from build123d import *

# Parameters (mm, degrees)
F0_R     = 21.2725
F1_DEPTH = 3.175
F2_R     = 21.2725
F3_DEPTH = 3.175
F4_R     = 11.43
F5_DEPTH = 0.889
F6_R     = 0.635


with BuildPart() as f1:
    # F0 (on Top) → F1 (new body)
    with BuildSketch(Plane.XY):
        Circle(F0_R)
    extrude(amount=-F1_DEPTH)

    # F2 (on face) → F3 (join)
    with BuildSketch(Plane(origin=(0, 0, -3.175), x_dir=(1, 0, 0), z_dir=(0, 0, -1))):
        Circle(F2_R)
    extrude(amount=F3_DEPTH)

    # F4 (on face) → F5 (join)
    with BuildSketch(Plane(origin=(0, 0, -6.35), x_dir=(1, 0, 0), z_dir=(0, 0, -1))):
        Circle(F4_R)
    extrude(amount=F5_DEPTH)

    # F6
    f6_edges = [f1.edges().sort_by_distance(p)[0] for p in [
        (-11.43, 0, -7.239),
    ]]
    fillet(f6_edges, radius=F6_R)


solid = f1.part
Geometry check sheet. Reference: the model listing, model coordinates, mm. A direction names the side the tool comes from. Coordinates: 2 decimals unless noted, no trailing zeros. Order: outer loops, then holes, each group sorted by start corner. A loop starts at its lowest first (then second) coordinate and runs counter-clockwise, first axis right, second up. Notation, with made-up numbers: (28, 30.25) -> (62, 30.25) arc R23 cw to (62, 47.25) -> close; hole circle Ø1 at (2, 25). An arc over 180 degrees is marked (long way). Use a Markdown table: item, result. Add a question column.
1. Cross-section at C-C (z = -3.5). Enter the section's corners in (x, y) (1 decimal).
2. Cross-section at D-D (x = -16.5). Enter the section's corners in (y, z).
3. Go/stop test with flat-tipped pins: pin 1 Ø1.5 at (x, z) = (8.5, -2.5) entering from -Y; pin 2 Ø2 at (y, z) = (5.5, -1.5) entering from -X; pin 3 Ø3 at (x, z) = (0.5, -1) entering from +Y. Record where each tip stops, or that it passes through.
4. Set-up check for faces 1 (the face through (9, 9, -6.35)), 2 (the face through (0, 0, 0)): record each of +Z, -Z, +X, -X, +Y, -Y from which the full face is reachable in a straight line by a thin tool's end or side.
5. Material ranges on L1, parallel to Z at x = -6.5, y = -17; L2, parallel to Y at x = -0.5, z = -4.75; L3, parallel to X at y = 10, z = -1.75, recorded low to high.
Filled sheet:
| question | item | result |
|---|---|---|
| 1 | outline | circle Ø42.5 at (0, 0) |
| 2 | outline | (-13.43, -6.35) -> (13.43, -6.35) -> (13.43, 0) -> (-13.43, 0) -> close |
| 3 | pin 1 | y = -19.81 |
| 3 | pin 2 | x = -20.79 |
| 3 | pin 3 | y = 21.27 |
| 4 | face 1 | -Z |
| 4 | face 2 | +Z, +X, -X, +Y, -Y |
| 5 | L1 | -6.35 to 0 |
| 5 | L2 | -21.27 to 21.27 |
| 5 | L3 | -18.78 to 18.78 |
